```python
from build123d import *

# Parameters (mm, degrees)
F0_W     = 65.532
F0_H     = 65.532
F1_DEPTH = 5.08
F2_W     = 60.706
F2_H     = 60.706
F3_DEPTH = 10.16
F4_R     = 2.54
F6_DEPTH = 1.27
F8_R     = 1.27


with BuildPart() as f1:
    # F0 (on Top) → F1 (new body)
    with BuildSketch(Plane.XY):
        Rectangle(F0_W, F0_H)
    extrude(amount=-F1_DEPTH)

    # F2 (on Top) → F3 (join)
    with BuildSketch(Plane.XY):
        Rectangle(F2_W, F2_H)
    extrude(amount=-F3_DEPTH)

    # F4
    f4_edges = [f1.edges().sort_by_distance(p)[0] for p in [
        (-30.353, 30.353, -7.62),
        (30.353, 30.353, -7.62),
        (30.353, -30.353, -7.62),
        (-30.353, -30.353, -7.62),
    ]]
    fillet(f4_edges, radius=F4_R)

    # F5 (on Right) → F6 (join)
    with BuildSketch(Plane.YZ):
        Polygon((-11.3400844857, 9.3340231106), (-11.3400844857, 0), (-6.5773450769, 0), (-6.5773450769, 5.1228902303), (0, 5.1228902303), (0, 9.3340231106), align=None)
        Polygon((11.3400844857, 9.3340231106), (0, 9.3340231106), (0, 5.1228902303), (6.5773450769, 5.1228902303), (6.5773450769, 0), (11.3400844857, 0), align=None)
    extrude(amount=F6_DEPTH)

    # F7: F1 across plane


with BuildPart() as f1_1:
    add(f1.part)
    add(f1.part.mirror(Plane.YZ))

    # F8
    f8_edges = [f1_1.edges().sort_by_distance(p)[0] for p in [
        (0, -11.340084, 9.334023),
        (0, 11.340084, 9.334023),
    ]]
    fillet(f8_edges, radius=F8_R)


solid = f1_1.part
```
Input: part model. Units: mm. Frame: model coordinates. A direction names the side the tool comes from. Round coordinates to 2 decimals unless told otherwise and drop trailing zeros. Loops run counter-clockwise (first coordinate to the right, second up) from the corner with the lowest first, then second, coordinate; pieces in that order, holes last.
1) Pin query (flat end, axial travel): pin 1 (3 mm diameter, centred on x = 0, z = 6, fed in from -Y); pin 2 (1.3 mm diameter, centred on x = 0, z = 5, fed in from +Y); pin 3 (2 mm diameter, centred on x = -20, z = -7.5, fed in from -Y). Return the tip coordinate at first contact, or that it passes through.
Ans:
pin 1: stops at y = -11.34
pin 2: stops at y = 11.34
pin 3: stops at y = -30.35
2) Section query B-B on z = 2.25. Return the cut outline in (x, y), plus the area to 3 significant figures.
Ans:
outline: (-1.27, -11.34) - (1.27, -11.34) - (1.27, -6.58) - (-1.27, -6.58) - close; (-1.27, 6.58) - (1.27, 6.58) - (1.27, 11.34) - (-1.27, 11.34) - close
area: 24.2 mm2
3) Section query A-A on y = 3. Return the cut outline in (x, z), plus the area to 3 significant figures.
Ans:
outline: (-32.77, -5.08) - (-30.35, -5.08) - (-30.35, -10.16) - (30.35, -10.16) - (30.35, -5.08) - (32.77, -5.08) - (32.77, 0) - (-32.77, 0) - close; (-1.27, 5.12) - (1.27, 5.12) - (1.27, 9.33) - (-1.27, 9.33) - close
area: 652 mm2
4) Set-up query: faces 5 (the cylindrical face through (29.63, 29.59, -7.66)), 6 (the flat face through (-3, -31, -5.08)), 7 (the flat face through (0, -11.34, 4)). Return all of +Z, -Z, +X, -X, +Y, -Y with unobstructed straight access to the full face (end or side cutting, diameter ignored); none if empty.
Ans:
face 5: -Z, +X, +Y
face 6: -Z
face 7: +Z, +X, -X, -Y
5) Material intervals for line 1 (Y direction, x = 0, z = 4); line 2 (Z direction, x = 0, y = 3); line 3 (Z direction, x = -27.5, y = 27), sorted ascending.
Ans:
line 1: y = -11.34 to -6.58, 6.58 to 11.34
line 2: z = -10.16 to 0, 5.12 to 9.33
line 3: z = -10.16 to 0
6) Section query C-C on x = -0.5. Return the cut outline in (y, z), plus the area to 3 significant figures.
Ans:
outline: (-32.77, -5.08) - (-30.35, -5.08) - (-30.35, -10.16) - (30.35, -10.16) - (30.35, -5.08) - (32.77, -5.08) - (32.77, 0) - (11.34, 0) - (11.34, 8.06) arc R1.27 ccw to (10.07, 9.33) - (-10.07, 9.33) arc R1.27 ccw to (-11.34, 8.06) - (-11.34, 0) - (-32.77, 0) - close; hole (-6.58, 0) - (6.58, 0) - (6.58, 5.12) - (-6.58, 5.12) - close
area: 785 mm2
7) Section query D-D on y = -21. Return the cut outline in (x, z).
Ans:
outline: (-32.77, -5.08) - (-30.35, -5.08) - (-30.35, -10.16) - (30.35, -10.16) - (30.35, -5.08) - (32.77, -5.08) - (32.77, 0) - (-32.77, 0) - close
8) Pull-direction query (Y, two-part tool) for faces 1 (the flat face through (0, -6.577, 3)), 2 (the flat face through (30.353, 0, -8)), 3 (the flat face through (0, 11.34, 4)), 4 (the cylindrical face through (-29.59, -29.63, -7.66)); classes: released by +Y, released by -Y, zero draft, split by the parting line, or undercut.
Ans:
face 1: undercut
face 2: zero draft
face 3: released by +Y
face 4: released by -Y
